```python
from build123d import *

# Parameters (mm, degrees)
SKETCH2_W                    = 41.275
SKETCH2_H                    = 81.28
BASE_FLANGE1_DEPTH           = 3.175
EDGE_FLANGE1_STRIP_W         = 14.7
EDGE_FLANGE1_STRIP_H         = 3.175
EDGE_FLANGE1_STRIP_CUT_DEPTH = 41.275
EDGE_FLANGE1_DEPTH           = 41.275
CUT_EXTRUDE1_REACH           = 124.133
SKETCH10_R                   = 5.08
CUT_EXTRUDE3_REACH           = 124.133
SKETCH12_R                   = 5.08


# Sheet-metal steps are written as plain solids
with BuildPart() as part:
    # Sketch2 → Base-Flange1 (new body)
    with BuildSketch(Plane(origin=(0, 0, 0), x_dir=(1, 0, 0), z_dir=(0, 1, 0))):
        with Locations((20.6375, 40.64)):
            Rectangle(SKETCH2_W, SKETCH2_H)
    extrude(amount=-BASE_FLANGE1_DEPTH)

    # Edge-Flange1 strip (across the edge) → Edge-Flange1 strip cut (cut)
    with BuildSketch(Plane(origin=(0, 0, 0), x_dir=(0, 0, -1), z_dir=(1, 0, 0))):
        with Locations((-6.35, -1.5875)):
            Rectangle(EDGE_FLANGE1_STRIP_W, EDGE_FLANGE1_STRIP_H)
    extrude(amount=EDGE_FLANGE1_STRIP_CUT_DEPTH, mode=Mode.SUBTRACT)

    # Edge-Flange1 section (across the edge) → Edge-Flange1 (add)
    with BuildSketch(Plane(origin=(0, 0, 0), x_dir=(0, 0, -1), z_dir=(1, 0, 0))):
        with BuildLine():
            Line((-3.175, 1), (-3.175, 81.28))
            Line((-3.175, 81.28), (0, 81.28))
            Line((0, 81.28), (0, 1))
            ThreePointArc((0, 1), (0.292893219, 0.292893219), (1, 0))
            Line((1, 0), (1, -3.175))
            ThreePointArc((1, -3.175), (-1.952170811, -1.952170811), (-3.175, 1))
        make_face()
    extrude(amount=EDGE_FLANGE1_DEPTH)

    # Sketch10 → Cut-Extrude1 (cut, up to next)
    with BuildSketch(Plane(origin=(0, 0, 0), x_dir=(-1, 0, 0), z_dir=(0, 0, -1)), mode=Mode.PRIVATE) as cut_extrude1_sk1:
        with Locations((-20.6375, 62.638675326)):
            Circle(SKETCH10_R)
    cut_extrude1_tool1 = extrude(cut_extrude1_sk1.sketch, amount=-CUT_EXTRUDE1_REACH, mode=Mode.PRIVATE) & part.part
    # Sketch10 → Cut-Extrude1 (cut, up to next)
    with BuildSketch(Plane(origin=(0, 0, 0), x_dir=(-1, 0, 0), z_dir=(0, 0, -1)), mode=Mode.PRIVATE) as cut_extrude1_sk2:
        with Locations((-20.6375, 16.918675326)):
            Circle(SKETCH10_R)
    cut_extrude1_tool2 = extrude(cut_extrude1_sk2.sketch, amount=-CUT_EXTRUDE1_REACH, mode=Mode.PRIVATE) & part.part
    add(cut_extrude1_tool1.solids().sort_by_distance((20.6375, 62.638675, 0))[0], mode=Mode.SUBTRACT)
    add(cut_extrude1_tool2.solids().sort_by_distance((20.6375, 16.918675, 0))[0], mode=Mode.SUBTRACT)

    # Sketch12 → Cut-Extrude3 (cut, up to next)
    with BuildSketch(Plane(origin=(0, 0, 0), x_dir=(1, 0, 0), z_dir=(0, 1, 0)), mode=Mode.PRIVATE) as cut_extrude3_sk1:
        with Locations(Location((20.359792254, 16.65462957, 0), (0, 0, 270))):
            Circle(SKETCH12_R)
    cut_extrude3_tool1 = extrude(cut_extrude3_sk1.sketch, amount=-CUT_EXTRUDE3_REACH, mode=Mode.PRIVATE) & part.part
    # Sketch12 → Cut-Extrude3 (cut, up to next)
    with BuildSketch(Plane(origin=(0, 0, 0), x_dir=(1, 0, 0), z_dir=(0, 1, 0)), mode=Mode.PRIVATE) as cut_extrude3_sk2:
        with Locations(Location((20.360011307, 62.374629569, 0), (0, 0, 270))):
            Circle(SKETCH12_R)
    cut_extrude3_tool2 = extrude(cut_extrude3_sk2.sketch, amount=-CUT_EXTRUDE3_REACH, mode=Mode.PRIVATE) & part.part
    add(cut_extrude3_tool1.solids().sort_by_distance((20.359792, 0, -16.65463))[0], mode=Mode.SUBTRACT)
    add(cut_extrude3_tool2.solids().sort_by_distance((20.360011, 0, -62.37463))[0], mode=Mode.SUBTRACT)


solid = part.part
```
Design review of the part built by this model. Coordinates are the model's own, in mm. A direction names the side the tool comes from. Coordinates: 2 decimals unless noted, no trailing zeros. Loops run counter-clockwise (first coordinate to the right, second up) from the corner with the lowest first, then second, coordinate; pieces in that order, holes last.
Q1. Tool access review of faces 1 (the face through (20, 42, 0)), 2 (the face through (0, 20, 1)): name each direction out of +Z, -Z, +X, -X, +Y, -Y from which nothing blocks a thin tool from reaching the whole face with its end or side.
Reported:
face 1: -Z, +X, -X, +Y
face 2: +Z, -Z, -X, +Y, -Y
Q2. We need section B-B on z = -60.5. State the section outline as (x, y) points (3 decimals), and give its area (3 significant figures).
Reported:
outline: (0, -3.175) - (15.639, -3.175) - (15.639, 0) - (0, 0) - close; (25.081, -3.175) - (41.275, -3.175) - (41.275, 0) - (25.081, 0) - close
area: 101 mm2
Q3. We need section A-A on y = 15.5. State the section outline as (x, z) points (3 decimals), and give its area (3 significant figures).
Reported:
outline: (0, 0) - (15.76, 0) - (15.76, 3.175) - (0, 3.175) - close; (25.515, 0) - (41.275, 0) - (41.275, 3.175) - (25.515, 3.175) - close
area: 100 mm2
Q4. We need section D-D on z = -46.5. State the section outline as (x, y) points (3 decimals).
Reported:
outline: (0, -3.175) - (41.275, -3.175) - (41.275, 0) - (0, 0) - close
Q5. The part is to be moulded in two halves that separate along Y. For faces 3 (the face through (20.349, -1.984, 1.92)), 4 (the face through (20, 0, -42)), 5 (the face through (21.299, 21.955, 1.565)), say which applies: +Y half, -Y half, draft (parallel to the pull), parting line (faces both ways), or undercut.
Reported:
face 3: -Y half
face 4: +Y half
face 5: undercut
Q6. For pin 1 (1 mm diameter, centred on x = 23.5, y = 71, fed in from -Z); pin 2 (12 mm diameter, centred on x = 29, z = -64, fed in from +Y), all flat-tipped, find the tip position at first contact; note any pin that passes through.
Reported:
pin 1: stops at z = 0
pin 2: stops at y = 0
Q7. To check wall thickness, follow line 1 (Z direction, x = 38, y = 57) (3 decimals); line 2 (Y direction, x = 14, z = -28.5) (3 decimals). State the ranges of each line that lie inside material, in increasing order.
Reported:
line 1: z = 0 to 3.175
line 2: y = -3.175 to 0
Q8. We need section C-C on x = 27.5. State the section outline as (y, z) points (3 decimals), and give its area (3 significant figures).
Reported:
outline: (-3.175, -81.28) - (0, -81.28) - (0, -1) arc R1 cw to (1, 0) - (81.28, 0) - (81.28, 3.175) - (1, 3.175) arc R4.175 ccw to (-3.175, -1) - close
area: 523 mm2
